```python
from build123d import *

# Parameters (mm, degrees)
SKETCH1_W           = 80.264
SKETCH1_H           = 48.006
SKETCH1_W_2         = 71.12
SKETCH1_H_2         = 38.862
BOSS_EXTRUDE1_DEPTH = 6.35
CUT_EXTRUDE2_DEPTH  = 48.191566333
FILLET1_R           = 2.54


with BuildPart() as part:
    # Sketch1 → Boss-Extrude1 (new body)
    # profile 1 of 2: a face of its own
    with BuildSketch(Plane.XY):
        Rectangle(SKETCH1_W, SKETCH1_H)
        Rectangle(SKETCH1_W_2, SKETCH1_H_2, mode=Mode.SUBTRACT)
    # profile 2 of 2: a face of its own
    with BuildSketch(Plane.XY):
        Rectangle(SKETCH1_W_2, SKETCH1_H_2)
    extrude(amount=BOSS_EXTRUDE1_DEPTH)

    # Sketch2 → Cut-Extrude2 (cut, through all)
    with BuildSketch(Plane.XY.offset(6.35)):
        with BuildLine():
            ThreePointArc((-33.459999882, 19.431), (-37.044924324, 20.915924324), (-35.56, 17.330999882))
            Line((-35.56, 17.330999882), (-35.56, 19.431))
            Line((-35.56, 19.431), (-33.459999882, 19.431))
        make_face()
        with BuildLine():
            Line((-35.56, 19.431), (-35.56, 17.330999882))
            ThreePointArc((-35.56, 17.330999882), (-34.075075676, 17.946075676), (-33.459999882, 19.431))
            Line((-33.459999882, 19.431), (-35.56, 19.431))
        make_face()
        with BuildLine():
            Line((-35.56, -17.330999882), (-35.56, -19.431))
            Line((-35.56, -19.431), (-33.459999882, -19.431))
            ThreePointArc((-33.459999882, -19.431), (-34.075075676, -17.946075676), (-35.56, -17.330999882))
        make_face()
        with BuildLine():
            Line((-33.459999882, -19.431), (-35.56, -19.431))
            Line((-35.56, -19.431), (-35.56, -17.330999882))
            ThreePointArc((-35.56, -17.330999882), (-37.044924324, -20.915924324), (-33.459999882, -19.431))
        make_face()
        with BuildLine():
            ThreePointArc((33.459999882, 19.431), (34.075075676, 17.946075676), (35.56, 17.330999882))
            Line((35.56, 17.330999882), (35.56, 19.431))
            Line((35.56, 19.431), (33.459999882, 19.431))
        make_face()
        with BuildLine():
            Line((35.56, 19.431), (35.56, 17.330999882))
            ThreePointArc((35.56, 17.330999882), (37.044924324, 17.946075676), (37.660000118, 19.431))
            ThreePointArc((37.660000118, 19.431), (35.56, 21.531000118), (33.459999882, 19.431))
            Line((33.459999882, 19.431), (35.56, 19.431))
        make_face()
        with BuildLine():
            ThreePointArc((35.56, -17.330999882), (34.075075676, -17.946075676), (33.459999882, -19.431))
            Line((33.459999882, -19.431), (35.56, -19.431))
            Line((35.56, -19.431), (35.56, -17.330999882))
        make_face()
        with BuildLine():
            Line((35.56, -19.431), (33.459999882, -19.431))
            ThreePointArc((33.459999882, -19.431), (35.56, -21.531000118), (37.660000118, -19.431))
            ThreePointArc((37.660000118, -19.431), (37.044924324, -17.946075676), (35.56, -17.330999882))
            Line((35.56, -17.330999882), (35.56, -19.431))
        make_face()
    extrude(amount=-CUT_EXTRUDE2_DEPTH, mode=Mode.SUBTRACT)

    # Fillet1
    fillet1_edges = [part.edges().sort_by_distance(p)[0] for p in [
        (-40.132, -24.003, 3.175),
        (-40.132, 24.003, 3.175),
        (40.132, 24.003, 3.175),
        (40.132, -24.003, 3.175),
    ]]
    fillet(fillet1_edges, radius=FILLET1_R)


solid = part.part
```
Design review of the part built by this model. Coordinates are the model's own, in mm. Give positions to 0.01 mm unless a question says otherwise; leave off trailing zeros. Order: outer loops, then holes, each group sorted by start corner. A loop starts at its lowest first (then second) coordinate and runs counter-clockwise, first axis right, second up. Notation, with made-up numbers: M 22.5,17.5 L 70.5,17.5 A10 cw 70.5,24.5 Z; hole C -34.5,-3.5 d3. An arc over 180 degrees is marked long. One line per question, with ' | ' between items. Start each with the question number.
Q1. For pin 1 Ø5 at (x, y) = (-35.56, -19.431) entering from -Z, flat-tipped, find the tip position at first contact; note if it passes through.
Q2. For L1, parallel to Y at x = -35.56, z = 2.75; L2, parallel to X at y = 19, z = 0.5; L3, parallel to X at y = -21, z = 5.25, list the stretches that pass through material, from the lowest coordinate up. Write a range as [from, to].
Q3. We need section A-A (z = 1.5). Write out the cut boundary in (x, y).
Returned:
1) pin 1: z = 0
2) L1: [-24, -21.53], [-17.33, 17.33], [21.53, 24] | L2: [-40.13, -37.62], [-33.5, 33.5], [37.62, 40.13] | L3: [-40.13, -36.96], [-34.16, 34.16], [36.96, 40.13]
3) outline: M -40.13,-21.46 A2.54 ccw -37.59,-24 L 37.59,-24 A2.54 ccw 40.13,-21.46 L 40.13,21.46 A2.54 ccw 37.59,24 L -37.59,24 A2.54 ccw -40.13,21.46 Z; hole C -35.56,-19.43 d4.2; hole C -35.56,19.43 d4.2; hole C 35.56,-19.43 d4.2; hole C 35.56,19.43 d4.2
